Here's how the part is built. I have some questions about the finished solid (model axes, mm). A direction names the side the tool comes from. Coordinates: 2 decimals unless noted, no trailing zeros. Write each loop counter-clockwise with the first axis right and the second up, starting at its lowest first coordinate (ties: lowest second). Pieces come first, ordered by that corner, then holes. Notation, with made-up numbers: M 2.5,10 L 20.5,10 A28 ccw 20.5,41 Z; hole C -19,-37 d6. An arc over 180 degrees is marked long. Use one line per item in the form item = value. Start each with the question number.
1. Thinking about a two-plate mould opening in Y: for faces 3 (the face through (6, 0, 0)), 4 (the face through (1.246, -1.262, 4.006)), 5 (the face through (1.72, -0.007, 1.642)), which applies, released by +Y, released by -Y, zero draft, split by the parting line, or undercut?
2. On a 3-axis mill with a long thin cutter (end or side, diameter ignored), from which of +Z, -Z, +X, -X, +Y, -Y can I reach the whole of each face in a straight line? I mean faces 1 (the face through (5.044, 1.774, 0.923)), 2 (the face through (1.72, 0.007, -1.642)). Say none if no direction works.
3. Please list where these lines run through material, in increasing order: line 1 along Z through (x, y) = (2.5, -0.75) (3 decimals); line 2 along Y through (x, z) = (1.4, -1.5) (3 decimals); line 3 along Z through (x, y) = (2.75, 1) (3 decimals). Write a range as [from, to].
4. I'm going to push flat-ended pins straight in: pin 1 Ø2 at (y, z) = (3, 1.5) entering from +X; pin 2 Ø2 at (x, z) = (4.5, -2.5) entering from +Y; pin 3 Ø5 at (y, z) = (-3, 2) entering from -X. Where does each tip first touch, or does it pass through?
5. I want a section at A-A, the plane x = 4.6. List the corners of the cut face in (y, z) for me.
from build123d import *

# Parameters (mm, degrees)
FILLET1_R    = 1
RECPAT_COUNT = 2
RECPAT_ANGLE = 90


with BuildPart() as part:
    # BodySke → Base-Revolve (revolve)
    with BuildSketch(Plane.XY, mode=Mode.PRIVATE) as base_revolve_sk:
        with BuildLine():
            Line((0, 0), (6, 0))
            Line((6, 0), (6, 2))
            Line((6, 2), (3.7, 2))
            Line((3.7, 2), (1.5, 4.2))
            Line((1.5, 4.2), (1, 4.2))
            ThreePointArc((1, 4.2), (0.253446079, 2.158703314), (0, 0))
        make_face()
    revolve(base_revolve_sk.sketch.rotate(Axis((-15.875, 0, 0), (1, 0, 0)), 90), axis=Axis((-15.875, 0, 0), (1, 0, 0)))

    # Fillet1
    fillet1_edges = [part.edges().sort_by_distance(p)[0] for p in [
        (3.7, 0, -2),
    ]]
    fillet(fillet1_edges, radius=FILLET1_R)

    # Sketch3 → Recess section 0
    with BuildSketch(Plane(origin=(0, 0, 0), x_dir=(0, 0, -1), z_dir=(1, 0, 0))):
        with BuildLine():
            Line((0.515, -2.5), (-0.515, -2.5))
            Line((-0.515, -2.5), (-0.515, 2.5))
            Line((-0.515, 2.5), (0.515, 2.5))
            Line((0.515, 2.5), (0.515, -2.5))
        make_face()
    # Sketch4 → Recess section 1
    with BuildSketch(Plane(origin=(3.1, 0, 0), x_dir=(0, 0, -1), z_dir=(1, 0, 0))):
        with BuildLine():
            Line((0.515, -0.954397274), (-0.515, -0.954397274))
            Line((-0.515, -0.954397274), (-0.515, 0.954397274))
            Line((-0.515, 0.954397274), (0.515, 0.954397274))
            Line((0.515, 0.954397274), (0.515, -0.954397274))
        make_face()
    recess = loft(mode=Mode.SUBTRACT)

    # RecPat: Recess ×2 about axis
    recpat_axis = Axis((0, 0, 0), (1, 0, 0))
    for i in range(1, RECPAT_COUNT):
        add(recess.rotate(recpat_axis, i * RECPAT_ANGLE / (RECPAT_COUNT - 1)), mode=Mode.SUBTRACT)

    # RecCorSke → RecessCore (revolve, cut)
    with BuildSketch(Plane.XY, mode=Mode.PRIVATE) as recesscore_sk:
        Polygon((0, 0), (0, 1.067773117), (3.1, 0.851), (3.376506661, 0), align=None)
    revolve(recesscore_sk.sketch.rotate(Axis((-3.175, 0, 0), (1, 0, 0)), 90), axis=Axis((-3.175, 0, 0), (1, 0, 0)), mode=Mode.SUBTRACT)


solid = part.part
Answer list:
q1.face_3 = zero draft
q1.face_4 = split by the parting line
q1.face_5 = undercut
q2.face_1 = +X
q2.face_2 = -X
q3.line_1 = [-3.111, -0.515], [0.515, 3.111]
q3.line_2 = [-3.923, -0.515], [0.515, 3.923]
q3.line_3 = [-2.775, -0.515], [0.515, 2.775]
q4.pin_1 = 3.35
q4.pin_2 = 1.32
q4.pin_3 = 0.07
q5.outline = C 0,0 d4
